Model file for the job. Use its own axes, mm. Coordinates: 2 decimals unless noted, no trailing zeros.
Q1. Drill centre lines: probe 1 along Z at (x, y) = (9.75, -249); probe 2 along X at (y, z) = (-190, 11); probe 3 along Z at (x, y) = (12, -460.5) (1 decimal). Where is each one in solid material? Low to high.
Q2. Pin check, flat tips, straight feed: P1, Ø1.5, axis at x = -14.5, y = -203.5, coming from the +Z side; P2, Ø0.6, axis at x = 14.5, y = -209.5, coming from the -Z side. Stop position of each tip, or through.
Q3. Band-saw the part on A-A, the plane y = -242.5. State how many separate pieces and enclosed holes the cut face has, plus the area to 3 significant figures.
from build123d import *

# Parameters (mm, degrees)
F0_R     = 2.45
F1_DEPTH = 460
F2_DEPTH = 100


# Not quite as in the source:
# - ends of sketch curves that miss each other by under 0.0002 mm in the source are joined


with BuildPart() as f1:
    # F0 (on Front) → F1 (new body)
    with BuildSketch(Plane.XZ):
        with BuildLine():
            Line((-3.1749674082, 15), (-12, 15))
            ThreePointArc((-12, 15), (-14.1213203436, 14.1213203436), (-15, 12))
            Line((-15, 12), (-15, 3.175))
            Line((-15, 3.175), (-13.0855346263, 3.175))
            ThreePointArc((-13.0855346263, 3.175), (-12.3835980145, 3.4627605788), (-12.0856407741, 4.1604300138))
            Line((-12.0856407741, 4.1604300138), (-12.0761692778, 4.8104300138))
            ThreePointArc((-12.0761692778, 4.8104300138), (-12.3638237087, 5.5269366118), (-13.0760631299, 5.825))
            Line((-13.0760631299, 5.825), (-13.5, 5.825))
            Line((-13.5, 5.825), (-13.5, 8.225))
            Line((-13.5, 8.225), (-9.8968845016, 8.225))
            ThreePointArc((-9.8968845016, 8.225), (-9.5279915195, 8.1544718757), (-9.2111331975, 7.9528359354))
            Line((-9.2111331975, 7.9528359354), (-5.4142486959, 4.3754933338))
            ThreePointArc((-5.4142486959, 4.3754933338), (-5.1819174045, 4.0440465354), (-5.1, 3.6476573984))
            Line((-5.1, 3.6476573984), (-5.1, -3.4999243287))
            ThreePointArc((-5.1, -3.4999243287), (-5.1782354607, -3.8876744211), (-5.4007002683, -4.2147528992))
            Line((-5.4007002683, -4.2147528992), (-9.2084959767, -7.9398285705))
            ThreePointArc((-9.2084959767, -7.9398285705), (-9.5301904718, -8.1509666761), (-9.9077957084, -8.225))
            Line((-9.9077957084, -8.225), (-13.5, -8.225))
            Line((-13.5, -8.225), (-13.5, -5.825))
            Line((-13.5, -5.825), (-13.0760631299, -5.825))
            ThreePointArc((-13.0760631299, -5.825), (-12.3638237087, -5.5269366118), (-12.0761692778, -4.8104300138))
            Line((-12.0761692778, -4.8104300138), (-12.0856407741, -4.1604300138))
            ThreePointArc((-12.0856407741, -4.1604300138), (-12.3835980145, -3.4627605788), (-13.0855346263, -3.175))
            Line((-13.0855346263, -3.175), (-15, -3.175))
            Line((-15, -3.175), (-15, -12))
            ThreePointArc((-15, -12), (-14.1213203436, -14.1213203436), (-12, -15))
            Line((-12, -15), (-3.175, -15))
            Line((-3.175, -15), (-3.175, -13.0855346263))
            ThreePointArc((-3.175, -13.0855346263), (-3.4627605788, -12.3835980145), (-4.1604300138, -12.0856407741))
            Line((-4.1604300138, -12.0856407741), (-4.8104300138, -12.0761692778))
            ThreePointArc((-4.8104300138, -12.0761692778), (-5.5269366118, -12.3638237087), (-5.825, -13.0760631299))
            Line((-5.825, -13.0760631299), (-5.825, -13.5))
            Line((-5.825, -13.5), (-8.225, -13.5))
            Line((-8.225, -13.5), (-8.225, -9.8968845016))
            ThreePointArc((-8.225, -9.8968845016), (-8.1544718757, -9.5279915195), (-7.9528359354, -9.2111331975))
            Line((-7.9528359354, -9.2111331975), (-4.3754933338, -5.4142486959))
            ThreePointArc((-4.3754933338, -5.4142486959), (-4.0440465354, -5.1819174045), (-3.6476573984, -5.1))
            Line((-3.6476573984, -5.1), (3.4999243287, -5.1))
            ThreePointArc((3.4999243287, -5.1), (3.8876744211, -5.1782354607), (4.2147528992, -5.4007002683))
            Line((4.2147528992, -5.4007002683), (7.9398285705, -9.2084959767))
            ThreePointArc((7.9398285705, -9.2084959767), (8.1509666761, -9.5301904718), (8.225, -9.9077957084))
            Line((8.225, -9.9077957084), (8.225, -13.5))
            Line((8.225, -13.5), (5.825, -13.5))
            Line((5.825, -13.5), (5.825, -13.0760631299))
            ThreePointArc((5.825, -13.0760631299), (5.5269366118, -12.3638237087), (4.8104300138, -12.0761692778))
            Line((4.8104300138, -12.0761692778), (4.1604300138, -12.0856407741))
            ThreePointArc((4.1604300138, -12.0856407741), (3.4627605788, -12.3835980145), (3.175, -13.0855346263))
            Line((3.175, -13.0855346263), (3.175, -15))
            Line((3.175, -15), (12, -15))
            ThreePointArc((12, -15), (14.1213203436, -14.1213203436), (15, -12))
            Line((15, -12), (15, -3.175))
            Line((15, -3.175), (13.0855346263, -3.175))
            ThreePointArc((13.0855346263, -3.175), (12.3835980145, -3.4627605788), (12.0856407741, -4.1604300138))
            Line((12.0856407741, -4.1604300138), (12.0761692778, -4.8104300138))
            ThreePointArc((12.0761692778, -4.8104300138), (12.3638237087, -5.5269366118), (13.0760631299, -5.825))
            Line((13.0760631299, -5.825), (13.5, -5.825))
            Line((13.5, -5.825), (13.5, -8.225))
            Line((13.5, -8.225), (9.9077957084, -8.225))
            ThreePointArc((9.9077957084, -8.225), (9.5301904718, -8.1509666761), (9.2084959767, -7.9398285705))
            Line((9.2084959767, -7.9398285705), (5.4007002683, -4.2147528992))
            ThreePointArc((5.4007002683, -4.2147528992), (5.1782354607, -3.8876744211), (5.1, -3.4999243287))
            Line((5.1, -3.4999243287), (5.1, 3.6476573984))
            ThreePointArc((5.1, 3.6476573984), (5.1819174045, 4.0440465354), (5.4142486959, 4.3754933338))
            Line((5.4142486959, 4.3754933338), (9.2111331975, 7.9528359354))
            ThreePointArc((9.2111331975, 7.9528359354), (9.5279915195, 8.1544718757), (9.8968845016, 8.225))
            Line((9.8968845016, 8.225), (13.5, 8.225))
            Line((13.5, 8.225), (13.5, 5.825))
            Line((13.5, 5.825), (13.0760631299, 5.825))
            ThreePointArc((13.0760631299, 5.825), (12.3638237087, 5.5269366118), (12.0761692778, 4.8104300138))
            Line((12.0761692778, 4.8104300138), (12.0856407741, 4.1604300138))
            ThreePointArc((12.0856407741, 4.1604300138), (12.3835980145, 3.4627605788), (13.0855346263, 3.175))
            Line((13.0855346263, 3.175), (15, 3.175))
            Line((15, 3.175), (15, 12))
            ThreePointArc((15, 12), (14.1213203436, 14.1213203436), (12, 15))
            Line((12, 15), (3.1750325918, 15))
            Line((3.1750325918, 15), (3.1750325918, 13.0854824722))
            ThreePointArc((3.1750325918, 13.0854824722), (3.4627931706, 12.3835458604), (4.1604626057, 12.0855886201))
            Line((4.1604626057, 12.0855886201), (4.8104626057, 12.0761171237))
            ThreePointArc((4.8104626057, 12.0761171237), (5.5269692036, 12.3637715546), (5.8250325918, 13.0760109758))
            Line((5.8250325918, 13.0760109758), (5.8250325918, 13.4999478459))
            Line((5.8250325918, 13.4999478459), (8.2250325918, 13.4999478459))
            Line((8.2250325918, 13.4999478459), (8.2250325918, 9.8968323476))
            ThreePointArc((8.2250325918, 9.8968323476), (8.1545044675, 9.5279393654), (7.9528685272, 9.2110810434))
            Line((7.9528685272, 9.2110810434), (4.3755259256, 5.4141965418))
            ThreePointArc((4.3755259256, 5.4141965418), (4.0440791272, 5.1818652505), (3.6476899902, 5.0999478459))
            Line((3.6476899902, 5.0999478459), (-3.4998917369, 5.0999478459))
            ThreePointArc((-3.4998917369, 5.0999478459), (-3.8876418293, 5.1781833067), (-4.2147203074, 5.4006481142))
            Line((-4.2147203074, 5.4006481142), (-7.9397959787, 9.2084438226))
            ThreePointArc((-7.9397959787, 9.2084438226), (-8.1509340843, 9.5301383177), (-8.2249674082, 9.9077435543))
            Line((-8.2249674082, 9.9077435543), (-8.2249674082, 13.4999478459))
            Line((-8.2249674082, 13.4999478459), (-5.8249674082, 13.4999478459))
            Line((-5.8249674082, 13.4999478459), (-5.8249674082, 13.0760109758))
            ThreePointArc((-5.8249674082, 13.0760109758), (-5.5269040199, 12.3637715546), (-4.810397422, 12.0761171237))
            Line((-4.810397422, 12.0761171237), (-4.160397422, 12.0855886201))
            ThreePointArc((-4.160397422, 12.0855886201), (-3.462727987, 12.3835458604), (-3.1749674082, 13.0854824722))
            Line((-3.1749674082, 13.0854824722), (-3.1749674082, 15))
        make_face()
        with BuildLine():
            Line((-13.5, -11.5), (-13.5, -9.7))
            Line((-13.5, -9.7), (-9.7, -9.7))
            Line((-9.7, -9.7), (-9.7, -13.5))
            Line((-9.7, -13.5), (-11.5, -13.5))
            ThreePointArc((-11.5, -13.5), (-12.9142135624, -12.9142135624), (-13.5, -11.5))
        make_face(mode=Mode.SUBTRACT)
        with BuildLine():
            Line((9.7, -9.7), (13.5, -9.7))
            Line((13.5, -9.7), (13.5, -11.5))
            ThreePointArc((13.5, -11.5), (12.9142135624, -12.9142135624), (11.5, -13.5))
            Line((11.5, -13.5), (9.7, -13.5))
            Line((9.7, -13.5), (9.7, -9.7))
        make_face(mode=Mode.SUBTRACT)
        with BuildLine():
            ThreePointArc((-13.5, 11.5), (-12.9142135624, 12.9142135624), (-11.5, 13.5))
            Line((-11.5, 13.5), (-9.7, 13.5))
            Line((-9.7, 13.5), (-9.7, 9.7))
            Line((-9.7, 9.7), (-13.5, 9.7))
            Line((-13.5, 9.7), (-13.5, 11.5))
        make_face(mode=Mode.SUBTRACT)
        Circle(F0_R, mode=Mode.SUBTRACT)
        with BuildLine():
            Line((9.7, 13.5), (11.5, 13.5))
            ThreePointArc((11.5, 13.5), (12.9142135624, 12.9142135624), (13.5, 11.5))
            Line((13.5, 11.5), (13.5, 9.7))
            Line((13.5, 9.7), (9.7, 9.7))
            Line((9.7, 9.7), (9.7, 13.5))
        make_face(mode=Mode.SUBTRACT)
    extrude(amount=F1_DEPTH)

    # F2 (add): a face of the model
    f2_faces = [f1.faces().sort_by_distance(p)[0] for p in [
        (5.2291627207, -460, 12.6659491494),
    ]]
    extrude(f2_faces, amount=F2_DEPTH)


solid = f1.part
Answer sheet:
1. probe 1: z = -15 to -13.5, -9.7 to -8.21, 8.21 to 9.7, 13.5 to 15
1. probe 2: x = -15 to -13.5, -9.7 to -8.22, 8.23 to 9.7, 13.5 to 15
1. probe 3: z = -15 to -13.4, -9.7 to -8.2, 8.2 to 9.7, 13.4 to 15
2. P1: stops at z = 14.44
2. P2: stops at z = -14.04
3. separate pieces: 1
3. enclosed holes: 5
3. area: 330 mm2
